The listing builds one solid part. Answer for the finished solid, in the listing's coordinates (mm). A direction names the side the tool comes from. Round coordinates to 2 decimals unless told otherwise and drop trailing zeros. Loops run counter-clockwise (first coordinate to the right, second up) from the corner with the lowest first, then second, coordinate; pieces in that order, holes last. Notation, with made-up numbers: M -32,-11.5 L 24,-11.5 A32 cw 24,24.5 Z; hole C 59,-25 d3. An arc over 180 degrees is marked long. Put each result on its own line as item: value. Start each with the question number.
(1) Straight lines are drawn through the part: line 1 (X direction, y = 0.1, z = 0); line 2 (X direction, y = 1.2, z = -25.5); line 3 (X direction, y = 2.35, z = -61.5). For each, find the intervals that lie inside material, in ascending order.
(2) Determine the mould class of faces 4 (the face through (-88.13, 1.48, -8.52)), 5 (the face through (88.28, 1.48, -8.7)), 6 (the face through (100.48, 1.52, 3.49)), 7 (the face through (0, 3, -61)) for opening direction X: released by +X, released by -X, zero draft, split by the parting line, or undercut.
(3) Section B-B, the plane z = -43 is taken. Determine the outline of the cut face in (x, y), then the cut area to 3 significant figures.
(4) Section C-C, the plane z = -85 is taken. Determine the outline of the cut face in (x, y).
(5) Which of the six approach directions +Z, -Z, +X, -X, +Y, -Y give full straight-line access (tool end or side, diameter ignored) to faces 1 (the face through (0, 0, -61)), 2 (the face through (-61.3, 1.5, 3.6)), 3 (the face through (-7.23, 1.48, -72.05))?
(6) Flat-ended cylindrical pins translate along their axes: P1, Ø1, axis at x = -74.5, y = 0.5, coming from the -Z side; P2, Ø0.7, axis at y = 2, z = -79.5, coming from the -X side; P3, Ø0.7, axis at x = -79, y = 1, coming from the -Z side; P4, Ø5, axis at x = 62, z = -86.5, coming from the -Y side. Find the tip coordinate at first contact, or state that the pin passes through.
(7) Section D-D, the plane x = -74 is taken. Determine the outline of the cut face in (y, z).
(8) Section A-A, the plane x = -9 is taken. Determine the outline of the cut face in (y, z), then the cut area to 3 significant figures.
```python
from build123d import *

# Parameters (mm, degrees)
SKETCH_1_R      = 1.6
EXTRUDE_1_DEPTH = 3
FILLET_1_R      = 5
FILLET_2_R      = 5


with BuildPart() as part:
    # 草图1 → 凸台-拉伸1 (new body)
    with BuildSketch(Plane(origin=(0, 0, 0), x_dir=(1, 0, 0), z_dir=(0, 1, 0))):
        with BuildLine():
            Line((-91.763881784, -5), (-64.576721038, -5))
            Line((-64.576721038, -5), (-59.560497815, -5))
            ThreePointArc((-59.560497815, -5), (0, 59.77), (59.560497815, -5))
            Line((59.560497815, -5), (64.576721038, -5))
            Line((64.576721038, -5), (91.763881784, -5))
            Line((91.763881784, -5), (101.777551781, -4.993991746))
            ThreePointArc((101.777551781, -4.993991746), (0, 101.9), (-101.777551781, -4.993991746))
            Line((-101.777551781, -4.993991746), (-91.763881784, -5))
        make_face()
        with Locations(Location((-96.9, 0, 0), (0, 0, 270))):
            Circle(SKETCH_1_R, mode=Mode.SUBTRACT)
        with Locations(Location((96.9, 0, 0), (0, 0, 270))):
            Circle(SKETCH_1_R, mode=Mode.SUBTRACT)
        with BuildLine():
            Line((-78.347003133, 5), (-80.514657051, 5))
            ThreePointArc((-80.514657051, 5), (-88.206048938, 8.609186997), (-90.345506507, 16.831501832))
            ThreePointArc((-90.345506507, 16.831501832), (-64.983113191, 64.983113191), (-16.831501832, 90.345506507))
            ThreePointArc((-16.831501832, 90.345506507), (-8.609186997, 88.206048938), (-5, 80.514657051))
            Line((-5, 80.514657051), (-5, 78.347003133))
            ThreePointArc((-5, 78.347003133), (-7.292728703, 71.975349568), (-13.119593832, 68.525390606))
            ThreePointArc((-13.119593832, 68.525390606), (-49.334840123, 49.334840123), (-68.525390606, 13.119593832))
            ThreePointArc((-68.525390606, 13.119593832), (-71.975349568, 7.292728703), (-78.347003133, 5))
        make_face(mode=Mode.SUBTRACT)
        with Locations(Location((-68.518647097, 68.518647097, 0), (0, 0, 270))):
            Circle(SKETCH_1_R, mode=Mode.SUBTRACT)
        with BuildLine():
            ThreePointArc((5, 80.514657051), (8.609186997, 88.206048938), (16.831501831, 90.345506507))
            ThreePointArc((16.831501831, 90.345506507), (64.983113191, 64.983113191), (90.345506507, 16.831501832))
            ThreePointArc((90.345506507, 16.831501832), (88.206048938, 8.609186997), (80.514657051, 5))
            Line((80.514657051, 5), (78.347003133, 5))
            ThreePointArc((78.347003133, 5), (71.975349568, 7.292728703), (68.525390606, 13.119593832))
            ThreePointArc((68.525390606, 13.119593832), (49.334840123, 49.334840123), (13.119593832, 68.525390606))
            ThreePointArc((13.119593832, 68.525390606), (7.292728703, 71.975349568), (5, 78.347003133))
            Line((5, 78.347003133), (5, 80.514657051))
        make_face(mode=Mode.SUBTRACT)
        with Locations(Location((0, 96.9, 0), (0, 0, 270))):
            Circle(SKETCH_1_R, mode=Mode.SUBTRACT)
        with Locations(Location((68.518647097, 68.518647097, 0), (0, 0, 270))):
            Circle(SKETCH_1_R, mode=Mode.SUBTRACT)
    extrude(amount=EXTRUDE_1_DEPTH)

    # 圆角1
    fillet_1_edges = [part.edges().sort_by_distance(p)[0] for p in [
        (-101.777551781, 1.5, 4.993991746),
        (101.777551781, 1.5, 4.993991746),
    ]]
    fillet(fillet_1_edges, radius=FILLET_1_R)

    # 圆角2
    fillet_2_edges = [part.edges().sort_by_distance(p)[0] for p in [
        (-59.560497815, 1.5, 5),
        (59.560497815, 1.5, 5),
    ]]
    fillet(fillet_2_edges, radius=FILLET_2_R)


solid = part.part
```
Recorded:
1. line 1: x = -101.9 to -98.5, -95.3 to -59.77, 59.77 to 95.3, 98.5 to 101.9
1. line 2: x = -98.66 to -88.29, -64.94 to -54.06, 54.06 to 64.94, 88.29 to 98.66
1. line 3: x = -81.25 to -68.29, -32.95 to 32.95, 68.29 to 81.25
2. face 4: undercut
2. face 5: undercut
2. face 6: released by +X
2. face 7: zero draft
3. outline: M -92.38,0 L -81.22,0 L -81.22,3 L -92.38,3 Z; M -54.94,0 L -41.51,0 L -41.51,3 L -54.94,3 Z; M 41.51,0 L 54.94,0 L 54.94,3 L 41.51,3 Z; M 81.22,0 L 92.38,0 L 92.38,3 L 81.22,3 Z
3. area: 148 mm²
4. outline: M -56.2,0 L -34.94,0 L -34.94,3 L -56.2,3 Z; M -6.06,0 L 6.06,0 L 6.06,3 L -6.06,3 Z; M 34.94,0 L 56.2,0 L 56.2,3 L 34.94,3 Z
5. face 1: +Z, -Z, +X, -X, -Y
5. face 2: +Z, +Y, -Y
5. face 3: +Y, -Y
6. P1: stops at z = -70.05
6. P2: stops at x = -64.18
6. P3: stops at z = -64.79
6. P4: passes through
7. outline: M 0,-70.05 L 3,-70.05 L 3,-54.49 L 0,-54.49 Z; M 0,-5.99 L 3,-5.99 L 3,5 L 0,5 Z
8. outline: M 0,-101.5 L 3,-101.5 L 3,-88.51 L 0,-88.51 Z; M 0,-70.35 L 3,-70.35 L 3,-59.09 L 0,-59.09 Z
8. area: 72.7 mm²
